Source: CAD feature listing. Evaluate the final solid. Frame: model axes, mm. A direction names the side the tool comes from. Round coordinates to 2 decimals unless told otherwise and drop trailing zeros. Write each loop counter-clockwise with the first axis right and the second up, starting at its lowest first coordinate (ties: lowest second). Pieces come first, ordered by that corner, then holes.
```python
from build123d import *

# Parameters (mm, degrees)
F0_W           = 13.375
F0_H           = 2
F1_DEPTH       = 25
F2_R           = 1.75
F3_DEPTH       = 2
F4_W           = 11.3
F4_H           = 7
F5_DEPTH       = 25
F5_DEPTH_BACK  = 11.5
F6_W           = 26
F6_H           = 6.5
F7_DEPTH       = 7
F9_DEPTH       = 7
F11_DEPTH      = 19.75
F11_DEPTH_BACK = 6.25
F12_T1_DEPTH   = 27.75
F12_T3_DEPTH   = 27.75
F12_T5_DEPTH   = 59
F14_DEPTH      = 15
F15_W          = 5.5
F15_H          = 5.5
F16_DEPTH      = 2
F17_DEPTH      = 2
F18_D          = 3


# Not quite as in the source:
# - a fillet or chamfer that OpenCascade refuses, or shapes differently, is made with other operations: its cross-section is extruded or revolved along the edge and cut away or added


with BuildPart() as f1:
    # F0 (on Right) → F1 (new body, symmetric)
    with BuildSketch(Plane.YZ):
        with Locations((6.6875, 1)):
            Rectangle(F0_W, F0_H)
    extrude(amount=F1_DEPTH, both=True)

    # F2 (on face) → F3 (cut, through all)
    with BuildSketch(Plane.XY.offset(2)):
        with Locations((-13, 4)):
            Circle(F2_R)
        with Locations((13, 4)):
            Circle(F2_R)
    extrude(amount=-F3_DEPTH, mode=Mode.SUBTRACT)

    # F4 (on Right) → F5 (join, two sides)
    with BuildSketch(Plane.YZ) as f5_sk:
        with Locations((-5.65, -1.5)):
            Rectangle(F4_W, F4_H)
    extrude(amount=F5_DEPTH)
    extrude(f5_sk.sketch, amount=-F5_DEPTH_BACK)

    # F6 (on face) → F7 (cut, through all)
    with BuildSketch(Plane(origin=(0, 0, -5), x_dir=(1, 0, 0), z_dir=(0, 0, -1))):
        with Locations((6.75, 8.05)):
            Rectangle(F6_W, F6_H)
    extrude(amount=-F7_DEPTH, mode=Mode.SUBTRACT)

    # F8 (on face) → F9 (cut, through all)
    with BuildSketch(Plane(origin=(0, 0, -5), x_dir=(1, 0, 0), z_dir=(0, 0, -1))):
        Polygon((13, 4.8), (0.5, 4.8), (2.5, 2.8), (11, 2.8), align=None)
    extrude(amount=-F9_DEPTH, mode=Mode.SUBTRACT)

    # F10 (on Right) → F11 (cut, two sides)
    with BuildSketch(Plane.YZ) as f11_sk:
        Polygon((-4.8, -5), (-2.8, -5), (-4.8, 7), align=None)
    extrude(amount=F11_DEPTH, mode=Mode.SUBTRACT)
    extrude(f11_sk.sketch, amount=-F11_DEPTH_BACK, mode=Mode.SUBTRACT)

    # F12: fillet of radius 4.5 on 3 edges, made by hand

    # F12_s2 → F12_t1 (cut)
    with BuildSketch(Plane.YZ.offset(-22.75)):
        with BuildLine():
            ThreePointArc((-6.8, -5), (-9.9819805153, -3.6819805153), (-11.3, -0.5))
            Line((-11.3, -0.5), (-11.3, -5))
            Line((-11.3, -5), (-6.8, -5))
        make_face()
    extrude(amount=F12_T1_DEPTH, mode=Mode.SUBTRACT)

    # F12_s4 → F12_t3 (cut)
    with BuildSketch(Plane.YZ.offset(8.5)):
        with BuildLine():
            ThreePointArc((-6.8, -5), (-9.9819805153, -3.6819805153), (-11.3, -0.5))
            Line((-11.3, -0.5), (-11.3, -5))
            Line((-11.3, -5), (-6.8, -5))
        make_face()
    extrude(amount=F12_T3_DEPTH, mode=Mode.SUBTRACT)

    # F12_s6 → F12_t5 (cut)
    with BuildSketch(Plane.YZ.offset(-22.75)):
        with BuildLine():
            ThreePointArc((0, -0.5), (-1.3180194847, -3.6819805153), (-4.5, -5))
            Line((-4.5, -5), (0, -5))
            Line((0, -5), (0, -0.5))
        make_face()
    extrude(amount=F12_T5_DEPTH, mode=Mode.SUBTRACT)

    # F13 (on face) → F14 (join)
    with BuildSketch(Plane.XY.offset(2)):
        Polygon((25, 0), (-11.5, 0), (-11.5, -11.3), (-6.25, -11.3), (-6.25, -3.9666666667), (1.3333333333, -3.9666666667), (2.5, -2.8), (11, -2.8), (12.1666666667, -3.9666666667), (19.75, -3.9666666667), (19.75, -11.3), (25, -11.3), align=None)
    extrude(amount=F14_DEPTH)

    # F15 (on face) → F16 (join)
    with BuildSketch(Plane(origin=(0, 0, 0), x_dir=(-1, 0, 0), z_dir=(0, 1, 0))):
        with Locations((-16.04918, 10.25)):
            Rectangle(F15_W, F15_H)
        with Locations((2.45082, 10.25)):
            Rectangle(F15_W, F15_H)
    extrude(amount=-F16_DEPTH)

    # F15 (on face) → F17 (cut)
    with BuildSketch(Plane(origin=(0, 0, 0), x_dir=(-1, 0, 0), z_dir=(0, 1, 0))):
        with Locations((-16.04918, 10.25)):
            Rectangle(F15_W, F15_H)
        with Locations((2.45082, 10.25)):
            Rectangle(F15_W, F15_H)
    extrude(amount=-F17_DEPTH, mode=Mode.SUBTRACT)

    # F18 (through all)
    with Locations(Plane(origin=(0, 0, 0), x_dir=(-1, 0, 0), z_dir=(0, 1, 0))):
        with Locations((2.45082, 10.25), (-16.04918, 10.25)):
            Hole(F18_D / 2)


solid = f1.part
```
Q1. Mould query, pull axis Z, two halves, no side actions, for faces 1 (the face through (16, -1, 13)), 2 (the face through (-12.19, 2.45, 1.01)), 3 (the face through (6.494, -0.786, -3.04)), 4 (the face through (-3.641, -2.997, 9.337)). Classes: pulls with the +Z half, pulls with the -Z half, needs draft (parallel to the pull), parting line crosses it, or undercut.
Q2. Section query C-C, the plane y = 4.75. Output: boundary loops of the cut face in (x, z), and give its area (3 significant figures).
Q3. Section query B-B, the plane z = 10.25. Output: boundary loops of the cut face in (x, y).
Q4. Pin query (flat end, axial travel): P1, Ø10.5, axis at x = -2, y = 8.5, coming from the -Z side; P2, Ø4.5, axis at x = -3.5, z = 10.5, coming from the +Y side; P3, Ø5.5, axis at y = -3.5, z = 5, coming from the -X side. Return the tip coordinate at first contact, or that it passes through.
Q5. Section query A-A, the plane x = -13. Output: boundary loops of the cut face in (y, z) (3 decimals), and give its area (4 significant figures).
Q6. Set-up query: faces 5 (the face through (0, 7, 0)), 6 (the face through (15.3, -3.4, -1.4)), 7 (the face through (-18, 0, 1)), 8 (the face through (17.3, -2, 9.1)), 9 (the face through (0, 7, 2)). Return all of +Z, -Z, +X, -X, +Y, -Y with unobstructed straight access to the full face (end or side cutting, diameter ignored); none if empty.
Q7. Line query: line 1 (Y direction, x = -13, z = 0.8) (3 decimals); line 2 (X direction, y = -8.5, z = 6); line 3 (Z direction, x = 15, y = 9). Output: solid intervals per line, ascending.
Q8. Section query D-D, the plane z = 3. Output: boundary loops of the cut face in (x, y).
Filled in:
1. face 1: undercut
1. face 2: needs draft
1. face 3: pulls with the -Z half
1. face 4: undercut
2. outline: (-25, 0) - (-14.58, 0) - (-14.58, 2) - (-25, 2) - close; (-11.42, 0) - (11.42, 0) - (11.42, 2) - (-11.42, 2) - close; (14.58, 0) - (25, 0) - (25, 2) - (14.58, 2) - close
2. area: 87.4 mm2
3. outline: (-11.5, -11.3) - (-6.25, -11.3) - (-6.25, -3.97) - (-3.95, -3.97) - (-3.95, -2) - (-5.2, -2) - (-5.2, 0) - (-11.5, 0) - close; (-0.95, -3.97) - (1.33, -3.97) - (2.5, -2.8) - (11, -2.8) - (12.17, -3.97) - (14.55, -3.97) - (14.55, -2) - (13.3, -2) - (13.3, 0) - (0.3, 0) - (0.3, -2) - (-0.95, -2) - close; (17.55, -3.97) - (19.75, -3.97) - (19.75, -11.3) - (25, -11.3) - (25, 0) - (18.8, 0) - (18.8, -2) - (17.55, -2) - close
4. P1: stops at z = 0
4. P2: stops at y = 0
4. P3: stops at x = -11.5
5. outline: (0, 0) - (2.25, 0) - (2.25, 2) - (0, 2) - close; (5.75, 0) - (13.375, 0) - (13.375, 2) - (5.75, 2) - close
5. area: 19.75 mm2
6. face 5: -Z, +X, -X, +Y
6. face 6: -Z, -Y
6. face 7: +Z, -Z, -X, -Y
6. face 8: +Y
6. face 9: +Z, +X, -X, +Y
7. line 1: y = 0 to 2.25, 5.75 to 13.375
7. line 2: x = -11.5 to -6.25, 19.75 to 25
7. line 3: z = 0 to 2
8. outline: (-11.5, -11.3) - (-6.25, -11.3) - (-6.25, -3.97) - (1.33, -3.97) - (2.5, -2.8) - (11, -2.8) - (12.17, -3.97) - (19.75, -3.97) - (19.75, -11.3) - (25, -11.3) - (25, 0) - (-11.5, 0) - close
